from build123d import *

# Parameters (mm, degrees)
BOSS_EXTRU_1_DEPTH      = 5
ESQUISSE2_R             = 3
ENL_V_MAT_EXTRU_1_DEPTH = 5
ESQUISSE3_W             = 200
ESQUISSE3_H             = 10
ENL_V_MAT_EXTRU_2_DEPTH = 10
ESQUISSE4_R             = 2
ENL_V_MAT_EXTRU_3_DEPTH = 297.858552176
ESQUISSE5_W             = 50
ESQUISSE5_H             = 35
ENL_V_MAT_EXTRU_4_DEPTH = 297.858552176
ESQUISSE6_R             = 2.6
ESQUISSE6_R_2           = 2.779338986
ESQUISSE6_R_3           = 2.697585155
ESQUISSE6_R_4           = 2.469314184
ENL_V_MAT_EXTRU_5_DEPTH = 297.858552176


with BuildPart() as part:
    # Esquisse1 → Boss.-Extru.1 (new body)
    with BuildSketch(Plane.XY):
        with BuildLine():
            Line((10, 0), (240, 0))
            ThreePointArc((240, 0), (247.071067812, -2.928932188), (250, -10))
            Line((250, -10), (250, -160))
            Line((250, -160), (0, -160))
            Line((0, -160), (0, -10))
            ThreePointArc((0, -10), (2.928932188, -2.928932188), (10, 0))
        make_face()
    extrude(amount=BOSS_EXTRU_1_DEPTH)

    # Esquisse2 → Enlèv. mat.-Extru.1 (cut)
    with BuildSketch(Plane.XY.offset(5)):
        with Locations((10, -5)):
            Circle(ESQUISSE2_R)
        with Locations(Location((240, -55, 0), (0, 0, 180))):
            Circle(ESQUISSE2_R)
        with Locations(Location((240, -5, 0), (0, 0, 180))):
            Circle(ESQUISSE2_R)
        with Locations((10, -70)):
            Circle(ESQUISSE2_R)
    extrude(amount=-ENL_V_MAT_EXTRU_1_DEPTH, mode=Mode.SUBTRACT)

    # Esquisse3 → Enlèv. mat.-Extru.2 (cut)
    with BuildSketch(Plane(origin=(0, 0, 0), x_dir=(-1, 0, 0), z_dir=(0, 0, -1))):
        with Locations((-125, -5)):
            Rectangle(ESQUISSE3_W, ESQUISSE3_H)
    extrude(amount=-ENL_V_MAT_EXTRU_2_DEPTH, mode=Mode.SUBTRACT)

    # Esquisse4 → Enlèv. mat.-Extru.3 (cut, through all)
    with BuildSketch(Plane(origin=(0, 0, 0), x_dir=(-1, 0, 0), z_dir=(0, 0, -1))):
        with Locations((-8.002599179, -19.132336536)):
            Circle(ESQUISSE4_R)
        with Locations((-72.047815248, -16.649941006)):
            Circle(ESQUISSE4_R)
    extrude(amount=-ENL_V_MAT_EXTRU_3_DEPTH, mode=Mode.SUBTRACT)

    # Esquisse5 → Enlèv. mat.-Extru.4 (cut, through all)
    with BuildSketch(Plane(origin=(0, 0, 0), x_dir=(-1, 0, 0), z_dir=(0, 0, -1))):
        with Locations((-125, -142.5)):
            Rectangle(ESQUISSE5_W, ESQUISSE5_H)
    extrude(amount=-ENL_V_MAT_EXTRU_4_DEPTH, mode=Mode.SUBTRACT)

    # Esquisse6 → Enlèv. mat.-Extru.5 (cut, through all)
    with BuildSketch(Plane.XY.offset(5)):
        with Locations((83.25, -109.8)):
            Circle(ESQUISSE6_R)
        with Locations((83.25, -98.5)):
            Circle(ESQUISSE6_R_2)
        with Locations((166.75, -109.8)):
            Circle(ESQUISSE6_R_3)
        with Locations((166.75, -98.5)):
            Circle(ESQUISSE6_R_4)
    extrude(amount=-ENL_V_MAT_EXTRU_5_DEPTH, mode=Mode.SUBTRACT)


solid = part.part
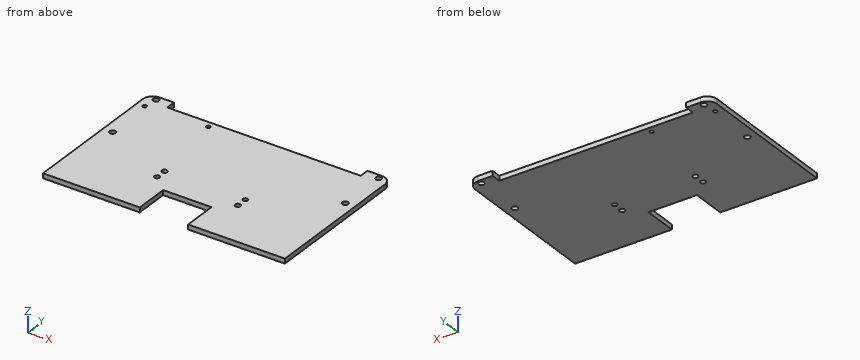
The listing builds one solid part. Answer for the finished solid, in the listing's coordinates (mm). Round coordinates to 2 decimals unless told otherwise and drop trailing zeros. Loops run counter-clockwise (first coordinate to the right, second up) from the corner with the lowest first, then second, coordinate; pieces in that order, holes last. Notation, with made-up numbers: M 19,85.5 L 32,85.5 A10 ccw 32,99.5 Z; hole C 78.5,50 d3. An arc over 180 degrees is marked long. Return JSON: item names as keys, results as strings.
Q1. Find section A-A, the plane y = -98.5. Determine the outline of the cut face in (x, z), plus the area to 3 significant figures.
Results list:
{"outline": "M 0,0 L 80.47,0 L 80.47,5 L 0,5 Z; M 86.03,0 L 164.28,0 L 164.28,5 L 86.03,5 Z; M 169.22,0 L 250,0 L 250,5 L 169.22,5 Z", "area": "1,200 mm2"}
Q2. Find section C-C, the plane x = 83.25. Determine the outline of the cut face in (y, z).
Results list:
{"outline": "M -160,0 L -112.4,0 L -112.4,5 L -160,5 Z; M -107.2,0 L -101.28,0 L -101.28,5 L -107.2,5 Z; M -95.72,0 L -10,0 L -10,5 L -95.72,5 Z"}
Q3. Find section D-D, the plane z = 2.45. State how many separate pieces and enclosed holes the cut face has, plus the area to 3 significant figures.
Results list:
{"separate pieces": "1", "enclosed holes": "10", "area": "36,000 mm2"}
Q4. Find the intervals of material crossed by line 1 along Y through (x, z) = (240, 1.05); line 2 along Y through (x, z) = (83.25, 3); line 3 along X through (y, z) = (-109, 4.15), in increasing order. Write a range as from..to.
Results list:
{"line 1": "y = -160..-58, -52..-8, -2..0", "line 2": "y = -160..-112.4, -107.2..-101.28, -95.72..-10", "line 3": "x = 0..80.78, 85.72..164.17, 169.33..250"}
Q5. Each of these flat-tipped pins is pushed along its axis until it touches: pin 1 Ø1.5 at (y, z) = (-6.5, 2) entering from -X; pin 2 Ø2 at (x, z) = (180.5, 2) entering from +Y; pin 3 Ø1.5 at (x, z) = (117.5, 3) entering from -Y. Where does it stop, or does it pass through?
Results list:
{"pin 1": "stops at x = 0.39", "pin 2": "stops at y = -10", "pin 3": "stops at y = -125"}
Q6. Find section B-B, the plane y = -55. Determine the outline of the cut face in (x, z), plus the area to 3 significant figures.
Results list:
{"outline": "M 0,0 L 237,0 L 237,5 L 0,5 Z; M 243,0 L 250,0 L 250,5 L 243,5 Z", "area": "1,220 mm2"}
